from build123d import *

# Parameters (mm, degrees)
F0_W     = 124
F0_H     = 77
F1_DEPTH = 4.9
F2_W     = 116.6
F2_H     = 69.6
F3_DEPTH = 3
F5_DEPTH = 9.8
F6_W     = 26
F6_H     = 3.7
F7_DEPTH = 4.9
F8_W     = 16
F8_H     = 0.7
F9_DEPTH = 25


with BuildPart() as f1:
    # F0 (on Top) → F1 (new body)
    with BuildSketch(Plane.XY):
        with Locations((62, 38.5)):
            Rectangle(F0_W, F0_H)
    extrude(amount=F1_DEPTH)

    # F2 (on face) → F3 (cut)
    with BuildSketch(Plane.XY.offset(4.9)):
        with Locations((62, 38.5)):
            Rectangle(F2_W, F2_H)
    extrude(amount=-F3_DEPTH, mode=Mode.SUBTRACT)

    # F4 (on Top) → F5 (join)
    with BuildSketch(Plane.XY):
        Polygon((51, -10), (51, 0), (49, 0), (49, -13), (55.25, -13), (55.25, -9.5), align=None)
        Polygon((68.75, -9.5), (68.75, -13), (75, -13), (75, 0), (73, 0), (73, -10), align=None)
    extrude(amount=F5_DEPTH)

    # F6 (on face) → F7 (join, through all)
    with BuildSketch(Plane.XY.offset(4.9)):
        with Locations((62, 1.85)):
            Rectangle(F6_W, F6_H)
    extrude(amount=F7_DEPTH)

    # F8 (on face) → F9 (cut)
    with BuildSketch(Plane.XY.offset(9.8)):
        with Locations((62, 0.35)):
            Rectangle(F8_W, F8_H)
    extrude(amount=-F9_DEPTH, mode=Mode.SUBTRACT)


solid = f1.part
Could you check a few things on this model? Use its own coordinates, in mm. A direction names the side the tool comes from. Give positions to 0.01 mm unless a question says otherwise; leave off trailing zeros. Order: outer loops, then holes, each group sorted by start corner. A loop starts at its lowest first (then second) coordinate and runs counter-clockwise, first axis right, second up. Notation, with made-up numbers: (-16, -32) - (-10, -32) arc R24 cw to (-10, 7) - close; hole circle Ø8 at (46, 17.5). An arc over 180 degrees is marked (long way). Return JSON: item names as keys, results as strings. Group by question number.
Q1. Thinking about a two-plate mould opening in Y: for faces 6 (the face through (120.3, 38, 3)), 7 (the face through (52, -13, 5)), 8 (the face through (61, 77, 2)), which applies, pulls with the +Y half, pulls with the -Y half, needs draft (parallel to the pull), parting line crosses it, or undercut?
Q2. Suppose I cut it at B-B, the plane x = 26.5. Please give me the cut outline in (y, z).
Q3. Which directions (+Z, -Z, +X, -X, +Y, -Y) give clear straight access to the entire face, cutting with the end or side of a thin tool? Please do faces 1 (the face through (62, 0.7, 5)), 2 (the face through (99, 0, 2)), 3 (the face through (3.7, 38, 3)), 4 (the face through (24, 0, 2)), 5 (the face through (55.25, -11, 5)).
Q4. Will these pins go through, and if not, where does the flat tip stop? pin 1 Ø4 at (x, z) = (96, 1.5) entering from -Y; pin 2 Ø3 at (y, z) = (-5.5, 2.5) entering from -X; pin 3 Ø1 at (x, y) = (23.5, 19.5) entering from +Z; pin 4 Ø8 at (x, y) = (83.5, 49) entering from -Z.
Q5. Suppose I cut it at A-A, the plane y = -6.5. Please give me the cut outline in (x, z), and give its area (3 significant figures).
Q6. Please list where these lines run through material, in increasing order: line 1 along Y through (x, z) = (71, 2.5); line 2 along X through (y, z) = (21, 4); line 3 along Y through (x, z) = (31, 4.25). Write a range as [from, to].
Q7. Suppose I cut it at C-C, the plane z = 6.5. Please give me the cut outline in (x, y), and give its area (3 significant figures).
Q8. Suppose I cut it at D-D, the plane y = 31. Please give me the cut outline in (x, z).
Resolved:
{
 "1": {"face 6": "undercut", "face 7": "pulls with the -Y half", "face 8": "pulls with the +Y half"},
 "2": {"outline": "(0, 0) - (77, 0) - (77, 4.9) - (73.3, 4.9) - (73.3, 1.9) - (3.7, 1.9) - (3.7, 4.9) - (0, 4.9) - close"},
 "3": {"face 1": "+Z, -Z", "face 2": "+Z, -Z, +X, -Y", "face 3": "+Z", "face 4": "+Z, -Z, -X, -Y", "face 5": "+Z, -Z, -Y"},
 "4": {"pin 1": "stops at y = 0", "pin 2": "stops at x = 49", "pin 3": "stops at z = 1.9", "pin 4": "stops at z = 0"},
 "5": {"outline": "(49, 0) - (51, 0) - (51, 9.8) - (49, 9.8) - close; (73, 0) - (75, 0) - (75, 9.8) - (73, 9.8) - close", "area": "39.2 mm2"},
 "6": {"line 1": "y = [-13, -9.76], [0, 3.7], [73.3, 77]", "line 2": "x = [0, 3.7], [120.3, 124]", "line 3": "y = [0, 3.7], [73.3, 77]"},
 "7": {"outline": "(49, -13) - (55.25, -13) - (55.25, -9.5) - (51, -10) - (51, 0) - (54, 0) - (54, 0.7) - (70, 0.7) - (70, 0) - (73, 0) - (73, -10) - (68.75, -9.5) - (68.75, -13) - (75, -13) - (75, 3.7) - (49, 3.7) - close", "area": "165 mm2"},
 "8": {"outline": "(0, 0) - (124, 0) - (124, 4.9) - (120.3, 4.9) - (120.3, 1.9) - (3.7, 1.9) - (3.7, 4.9) - (0, 4.9) - close"}
}
